Check sheet for the modelled part. Datum: model origin and axes. Units: mm. Face numbers are marked on the shaded views. A direction names the side the tool comes from. Coordinates: 2 decimals unless noted, no trailing zeros. Loops run counter-clockwise (first coordinate to the right, second up) from the corner with the lowest first, then second, coordinate; pieces in that order, holes last.
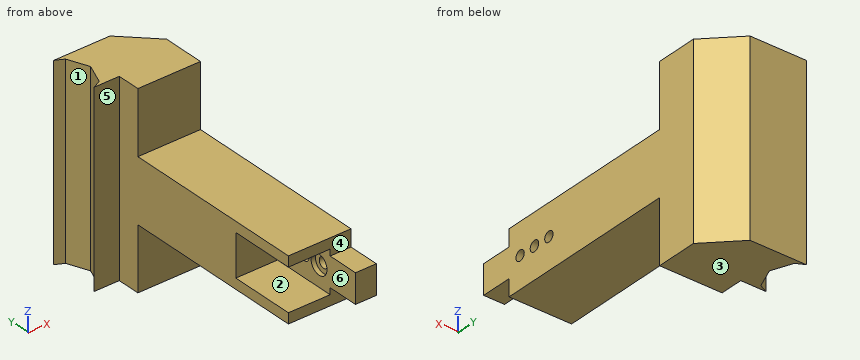
Autodesk Inventor part; units mm, degrees
ref_plane "Work Plane1" through (0, 0, -15) normal (0, 0, 1) x (1, 0, 0)
ref_plane "YZ Plane" through (0, 0, 0) normal (1, 0, 0) x (0, 1, 0)
ref_plane "XZ Plane" through (0, 0, 0) normal (0, 1, 0) x (-1, 0, 0)
sketch "Sketch1" plane through (0, 0, 0) normal (0, 0, 1) x (1, 0, 0)
  line L0 (0, 0) -> (25, 0)
  line L1 (25, 0) -> (25, 40)
  line L2 (25, 40) -> (0, 40)
  line L3 (0, 40) -> (0, 0)
  dimension "d1" = 25
  dimension "d2" = 40
  dimension "d3" = 25
extrude "Extrusion1" add sketch "Sketch1" against normal blind 30
sketch "Sketch2" plane through (25, 0, 0) normal (1, 0, 0) x (0, 0, -1)
  line L0 (0, 0) -> (30, 0)
  circle A0 centre (15, 6.56) radius 2.46
extrude "Extrusion2" cut sketch "Sketch2" against normal blind 30
sketch "Sketch3" plane through (0, 0, 0) normal (-1, 0, 0) x (0, 0, 1)
  line L0 (0, 0) -> (-30, 0)
  line L1 (-25.05, 0) -> (-4.95, 0)
  line L2 (-4.95, 0) -> (-4.95, 33.12)
  line L3 (-4.95, 33.12) -> (-25.05, 33.12)
  line L4 (-25.05, 33.12) -> (-25.05, 0)
  dimension "d11" = 20.1
extrude "Extrusion3" cut sketch "Sketch3" against normal blind 20
sketch "Sketch4" plane through (0, 0, 0) normal (0, -1, 0) x (1, 0, 0)
  line L0 (20, -4.95) -> (20, -25.05)
  line L1 (20, -15) -> (25, -15)
  line L2 (25, 0) -> (25, -30)
  line L3 (20, -8.025) -> (25, -8.025)
  line L4 (25, -8.025) -> (25, -21.975)
  line L5 (25, -21.975) -> (20, -21.975)
  line L6 (20, -21.975) -> (20, -8.025)
  line L7 (20, -8.025) -> (25, -21.975) construction
  line L8 (25, -8.025) -> (20, -21.975) construction
  line L9 (25, -12.54) -> (25, -17.46)
  point P0 (0, 0)
  point P1 (22.5, -15)
  dimension "d14" = 13.95
extrude "Extrusion4" add sketch "Sketch4" along normal blind 15
sketch "Sketch5" plane through (20, 0, 0) normal (-1, 0, 0) x (0, 0, 1)
  circle A0 centre (-15, 6.56) radius 2.46
  circle A1 centre (-15, 6.56) radius 4.7025
  circle A2 centre (-15, 6.56) radius 2.46
  circle A3 centre (-15, 6.56) radius 2.46
  point P0 (0, 0)
  dimension "d17" = 9.405
extrude "Extrusion5" cut sketch "Sketch5" against normal blind 2.1
sketch "Sketch6" plane through (25, 0, 0) normal (1, 0, 0) x (0, 0, -1)
  circle A0 centre (15, 6.56) radius 4.7025
  line L0 (15, 6.56) -> (15, 23.56)
  circle A1 centre (15, 23.56) radius 2.46
  point P0 (0, 0)
  dimension "d20" = 17
  dimension "d21" = 4.92
extrude "Extrusion6" cut sketch "Sketch6" against normal blind 10 contours A1
sketch "Sketch7" plane through (20, 0, 0) normal (-1, 0, 0) x (0, 0, 1)
  circle A0 centre (-15, 23.56) radius 2.46
  circle A1 centre (-15, 23.56) radius 4.7025
  point P0 (0, 0)
  dimension "d24" = 9.405
extrude "Extrusion7" cut sketch "Sketch7" against normal blind 2.1
sketch "Sketch9" plane through (25, 0, 0) normal (1, 0, 0) x (0, 0, -1)
  circle A0 centre (15, 6.56) radius 2.46
  circle A1 centre (15, 6.56) radius 2.46
  circle A2 centre (15, 23.56) radius 2.46
  circle A3 centre (15, 23.56) radius 2.46
  line L0 (30, 40) -> (30, 0)
  line L1 (30, 0) -> (30, 40)
  line L2 (30, 40) -> (0, 40)
  line L3 (0, 40) -> (0, 0)
  line L4 (0, 0) -> (8.025, 0)
  line L5 (21.975, 0) -> (21.975, -15)
  line L6 (21.975, -15) -> (8.025, -15)
  line L7 (8.025, -15) -> (8.025, 0)
  line L8 (0, 0) -> (8.025, 0)
  line L9 (21.975, 0) -> (30, 0)
extrude "Extrusion8" add sketch "Sketch9" along normal blind 5
sketch "Sketch10" plane through (0, 40, 0) normal (0, 1, 0) x (1, 0, 0)
  line L0 (0, 30) -> (30, 30)
  line L1 (30, 0) -> (0, 0)
  line L2 (0, 30) -> (30, 30)
  line L3 (30, 30) -> (30, 0)
  line L4 (30, 0) -> (0, 0)
  line L5 (0, 0) -> (0, 30)
extrude "Extrusion9" add sketch "Sketch10" along normal blind 30
sketch "Sketch12" plane through (30, 0, 0) normal (1, 0, 0) x (0, 0, -1)
  circle A0 centre (15, 6.56) radius 2.46
  line L0 (15, 6.56) -> (15, 15.06)
  circle A1 centre (15, 15.06) radius 2.525
  point P0 (0, 0)
  dimension "d31" = 8.5
  dimension "d33" = 5.05
extrude "Extrusion10" cut sketch "Sketch12" against normal blind 30 contours A1
sketch "Sketch14" plane through (0, 0, 0) normal (0, 0, 1) x (1, 0, 0)
  line L0 (30, 70) -> (0, 70)
  line L1 (0, 70) -> (0, 85)
  line L2 (30, 0) -> (30, 70)
  line L3 (30, 109) -> (30, 70)
  line L4 (30, 105) -> (30, 100)
  line L5 (-12, 124) -> (15, 124)
  line L6 (-8, 122) -> (-12, 124)
  line L7 (-8, 122) -> (-4, 112)
  line L8 (-8, 102) -> (-12, 100)
  line L9 (-8, 102) -> (-4, 112)
  line L10 (30, 109) -> (15, 124)
  line L11 (0, 85) -> (0, 100)
  line L12 (0, 100) -> (-12, 100)
  point P0 (0, 0)
  dimension "d69" = 12
extrude "Extrusion12" add sketch "Sketch14" against normal blind 30
sketch "Sketch15" plane through (0, 0, -25.05) normal (-1, 0, 0) x (0, 0, 1)
  line L0 (0, 33.12) -> (20.1, 33.12)
  line L1 (20.1, 33.12) -> (20.1, 0)
  line L2 (0, 33.12) -> (20.1, 33.12)
  line L3 (20.1, 33.12) -> (20.1, 31.1)
  line L4 (20.1, 31.1) -> (0, 31.1)
  line L5 (0, 31.1) -> (0, 33.12)
  point P0 (25.05, 0)
  dimension "d57" = 2.02
extrude "Extrusion13" add sketch "Sketch15" against normal blind 20
sketch "Sketch19" plane through (0, 0, 0) normal (0, 0, 1) x (1, 0, 0)
  line L0 (0, 100) -> (-12, 100)
  line L1 (0, 100) -> (-12, 100)
  line L2 (-12, 100) -> (-8, 102)
  line L3 (-12, 100) -> (-8, 102)
  line L4 (-8, 102) -> (-4, 112)
  line L5 (-8, 102) -> (-4, 112)
  line L6 (-4, 112) -> (-8, 122)
  line L7 (-4, 112) -> (-8, 122)
  line L8 (-8, 122) -> (-12, 124)
  line L9 (-8, 122) -> (-12, 124)
  line L10 (-12, 124) -> (15, 124)
  line L11 (-12, 124) -> (15, 124)
  line L12 (15, 124) -> (30, 109)
  line L13 (15, 124) -> (30, 109)
  line L14 (30, 109) -> (30, 89)
  line L15 (30, 89) -> (0, 89)
  line L16 (0, 89) -> (0, 100)
  point P0 (0, 0)
  dimension "d71" = 20
  dimension "d72" = 30
extrude "Extrusion14" add sketch "Sketch19" along normal blind 30
ref_plane "Work Plane1" through (0, 0, -15) normal (0, 0, 1) x (1, 0, 0)
mirror "Mirror1" about plane through (0, 0, -15) normal (0, 0, 1) of "Extrusion14"
properties part number "rec_b_20mm_x_90mm"
1) Depth check by flat-ended pin: pin 1 (4 mm diameter, centred on x = 18.5, z = -45, fed in from -Y); pin 2 (7.5 mm diameter, centred on y = 6.56, z = -15, fed in from -X); pin 3 (9 mm diameter, centred on x = 20.5, y = 35.5, fed in from -Z). Enter the tip coordinate at first touch or a pass-through.
Answer sheet:
pin 1: stops at y = 89
pin 2: stops at x = 22.1
pin 3: stops at z = -30
2) Mould release check, pull along Z, two halves, no side actions. Record for the marked faces 1, 2 and 3: +Z half, -Z half, draft (parallel to the pull), parting line (faces both ways), or undercut.
Answer sheet:
face 1: draft
face 2: undercut
face 3: -Z half
3) Set-up check for the marked faces 4, 5 and 6: record each of +Z, -Z, +X, -X, +Y, -Y from which the full face is reachable in a straight line by a thin tool's end or side.
Answer sheet:
face 4: +Z, +X, -X, -Y
face 5: +Z, -Z, -X, -Y
face 6: -X, -Y
4) Section check D-D on z = -38. Enter the section's corners in (x, y).
Answer sheet:
outline: (-12, 100) - (0, 100) - (0, 89) - (30, 89) - (30, 109) - (15, 124) - (-12, 124) - (-8, 122) - (-4, 112) - (-8, 102) - close
5) Scan lines: line 1 (Z direction, x = 24, y = 15); line 2 (Y direction, x = 21.3, z = -15) (1 decimal); line 3 (Y direction, x = 21.2, z = -15) (1 decimal). Record each from-to range of solid material in increasing order.
Answer sheet:
line 1: z = -30 to -17.52, -12.48 to 0
line 2: y = -15 to 1.9, 11.3 to 12.5, 17.6 to 18.9, 28.3 to 117.7
line 3: y = -15 to 1.9, 11.3 to 12.5, 17.6 to 18.9, 28.3 to 117.8
6) Section check C-C on x = 27.5. Enter the section's corners in (y, z) (3 decimals).
Answer sheet:
outline: (-15, -21.975) - (0, -21.975) - (0, -30) - (89, -30) - (89, -60) - (111.5, -60) - (111.5, 30) - (89, 30) - (89, 0) - (0, 0) - (0, -8.025) - (-15, -8.025) - close; hole circle Ø4.92 at (6.56, -15); hole circle Ø5.05 at (15.06, -15); hole circle Ø4.92 at (23.56, -15)
7) Section check B-B on y = 6.56. Enter the section's corners in (x, z).
Answer sheet:
outline: (0, -30) - (30, -30) - (30, -17.46) - (22.1, -17.46) - (22.1, -19.7) - (20, -19.7) - (20, -25.05) - (0, -25.05) - close; (0, -4.95) - (20, -4.95) - (20, -10.3) - (22.1, -10.3) - (22.1, -12.54) - (30, -12.54) - (30, 0) - (0, 0) - close
8) Section check A-A on z = -15. Give the number of separate pieces and of enclosed holes in the cut face, plus the area to 3 significant figures.
Answer sheet:
separate pieces: 4
enclosed holes: 0
area: 3,130 mm2
